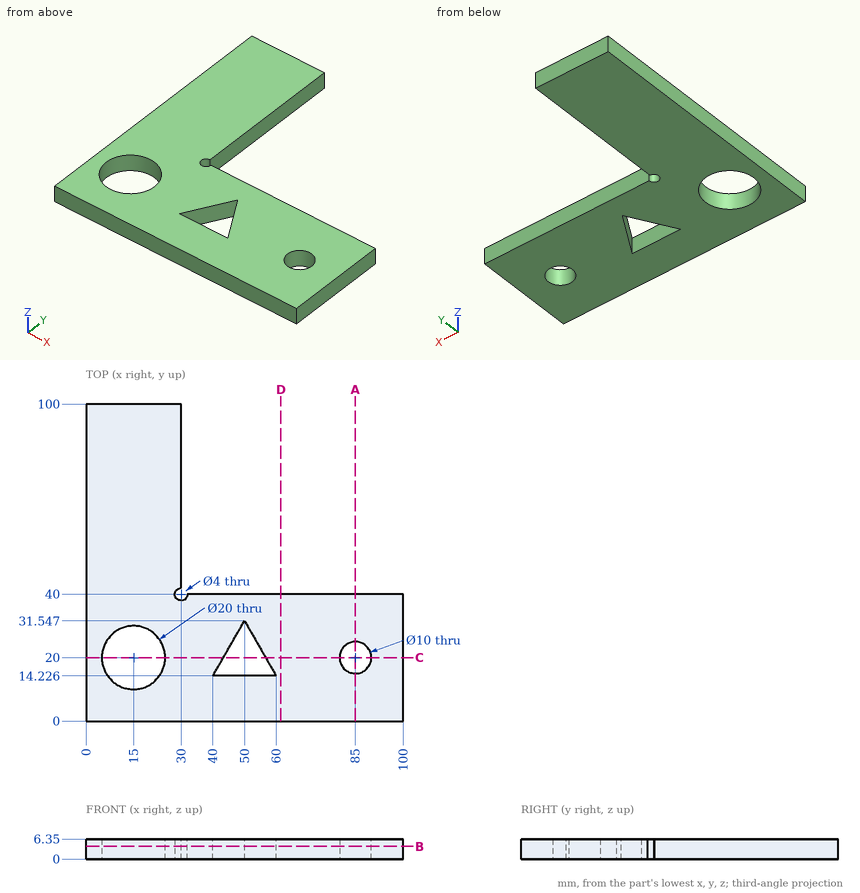
Print and shaded views of the part. All mm, measured from the part's lowest x, y and z. Give positions to 0.01 mm unless a question says otherwise; leave off trailing zeros. Loops run counter-clockwise (first coordinate to the right, second up) from the corner with the lowest first, then second, coordinate; pieces in that order, holes last.
1) Saw through at A-A (x = 85). Write the cut outline in (y, z).
2) Saw through at D-D (x = 61.5). Write the cut outline in (y, z), plus the area to 3 significant figures.
3) Saw through at C-C (y = 20). Write the cut outline in (x, z).
4) Saw through at B-B (z = 4). Write the cut outline in (x, y).
5) Wall check: line 1 (Y direction, x = 15, z = 4.25); line 2 (Y direction, x = 85, z = 1.5); line 3 (Y direction, x = 78, z = 6). Give the ranges that are in metal, low to high.
6) Flat gauge pins, fed straight in: pin 1 Ø2.5 at (x, y) = (30, 40) entering from -Z; pin 2 Ø3 at (x, z) = (67.5, 4) entering from +Y. Where does each tip first touch, or does it go through?
Answer block:
1. outline: (0, 0) - (15, 0) - (15, 6.35) - (0, 6.35) - close; (25, 0) - (40, 0) - (40, 6.35) - (25, 6.35) - close
2. outline: (0, 0) - (40, 0) - (40, 6.35) - (0, 6.35) - close
2. area: 254 mm2
3. outline: (0, 0) - (5, 0) - (5, 6.35) - (0, 6.35) - close; (25, 0) - (43.33, 0) - (43.33, 6.35) - (25, 6.35) - close; (56.67, 0) - (80, 0) - (80, 6.35) - (56.67, 6.35) - close; (90, 0) - (100, 0) - (100, 6.35) - (90, 6.35) - close
4. outline: (0, 0) - (100, 0) - (100, 40) - (32, 40) arc R2 cw (long way) to (30, 42) - (30, 100) - (0, 100) - close; hole circle Ø20 at (15, 20); hole (40, 14.23) - (60, 14.23) - (50, 31.55) - close; hole circle Ø10 at (85, 20)
5. line 1: y = 0 to 10, 30 to 100
5. line 2: y = 0 to 15, 25 to 40
5. line 3: y = 0 to 40
6. pin 1: passes through
6. pin 2: stops at y = 40
